For this review, use the dimensioned drawing (mm, ordinates from the lowest corner) and the shaded views. A direction names the side the tool comes from. Coordinates: 2 decimals unless noted, no trailing zeros. Write each loop counter-clockwise with the first axis right and the second up, starting at its lowest first coordinate (ties: lowest second). Pieces come first, ordered by that corner, then holes. Notation, with made-up numbers: (-12.5, 64.5) - (29.5, 64.5) arc R18 ccw to (29.5, 78.5) - close; hole circle Ø11 at (-18, 68). An arc over 180 degrees is marked (long way). Use one line per item in the form item = value. Start each with the question number.
1) Insertion check: P1, Ø1.6, axis at y = 4, z = 1.5, coming from the -X side; P2, Ø0.6, axis at x = 10.5, z = 1.5, coming from the -Y side (3 decimals); P3, Ø1.6, axis at y = 3, z = 1, coming from the +X side. Each pin has a flat end and moves straight along its axis. Give the tip position at first contact, or say it passes through.
2) We need section A-A (z = 1.5). Give the boundary of the cut face in (x, y) (3 decimals), plus the area to 4 significant figures.
3) We need section B-B (x = 14.75). Give the boundary of the cut face in (y, z), plus the area to 4 significant figures.
4) We need section C-C (y = 6.25). Give the boundary of the cut face in (x, z), plus the area to 3 significant figures.
5) Tool access review of the marked faces 1, 2 and 3: name each direction out of +Z, -Z, +X, -X, +Y, -Y from which nothing blocks a thin tool from reaching the whole face with its end or side.
6) We need section D-D (z = 6.5). Give the boundary of the cut face in (x, y).
7) For L1, parallel to X at y = 5.25, z = 6.5; L2, parallel to X at y = 5.5, z = 5.5; L3, parallel to Z at x = 14.75, y = 4.75, list the stretches that pass through material, from the lowest coordinate up. Write a range as from..to.
8) Mouldability with a two-part tool opening along X and no side actions: class the marked faces 4, 5, 6 and 7 as pulls with the +X half, pulls with the -X half, needs draft (parallel to the pull), parting line crosses it, or undercut.
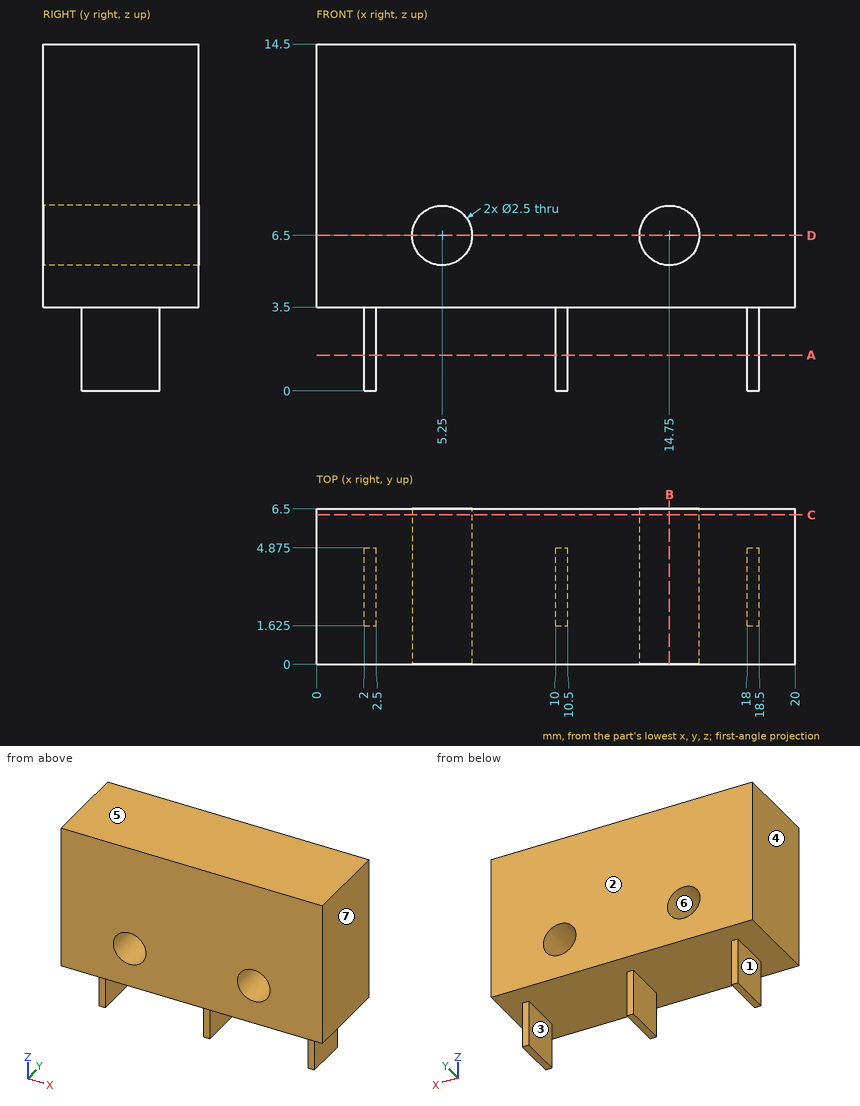
Determined:
q1.P1 = 2
q1.P2 = 1.625
q1.P3 = 18.5
q2.outline = (2, 1.625) - (2.5, 1.625) - (2.5, 4.875) - (2, 4.875) - close; (10, 1.625) - (10.5, 1.625) - (10.5, 4.875) - (10, 4.875) - close; (18, 1.625) - (18.5, 1.625) - (18.5, 4.875) - (18, 4.875) - close
q2.area = 4.875 mm²
q3.outline = (0, 3.5) - (6.5, 3.5) - (6.5, 5.25) - (0, 5.25) - close; (0, 7.75) - (6.5, 7.75) - (6.5, 14.5) - (0, 14.5) - close
q3.area = 55.25 mm²
q4.outline = (0, 3.5) - (20, 3.5) - (20, 14.5) - (0, 14.5) - close; hole circle Ø2.5 at (5.25, 6.5); hole circle Ø2.5 at (14.75, 6.5)
q4.area = 210 mm²
q5.face_1 = -Z, -X, +Y, -Y
q5.face_2 = +Z, -Z, +X, -X, +Y
q5.face_3 = -Z, +Y, -Y
q6.outline = (0, 0) - (4, 0) - (4, 6.5) - (0, 6.5) - close; (6.5, 0) - (13.5, 0) - (13.5, 6.5) - (6.5, 6.5) - close; (16, 0) - (20, 0) - (20, 6.5) - (16, 6.5) - close
q7.L1 = 0..4, 6.5..13.5, 16..20
q7.L2 = 0..4.5, 6..14, 15.5..20
q7.L3 = 3.5..5.25, 7.75..14.5
q8.face_4 = pulls with the -X half
q8.face_5 = needs draft
q8.face_6 = undercut
q8.face_7 = pulls with the +X half
